from build123d import *

# Parameters (mm, degrees)
SKETCH3_R           = 2
BOSS_EXTRUDE1_DEPTH = 2.54
FILLET1_R           = 1
BOSS_EXTRUDE2_START = -2.54
BOSS_EXTRUDE2_DEPTH = 8.15
CUT_EXTRUDE1_DEPTH  = 68.045951128
CUT_EXTRUDE2_REACH  = 68.573
CUT_EXTRUDE3_REACH  = 68.573


with BuildPart() as part:
    # Sketch3 → Boss-Extrude1 (new body)
    with BuildSketch(Plane(origin=(0, 0, 0), x_dir=(1, 0, 0), z_dir=(0, 1, 0))):
        with BuildLine():
            Line((-10.5, 12.675), (-14.80167643, 18.402233616))
            ThreePointArc((-14.80167643, 18.402233616), (-17.462309014, 19.963696306), (-20.442771336, 19.167470316))
            Line((-20.442771336, 19.167470316), (-26.332078502, 14.625602737))
            ThreePointArc((-26.332078502, 14.625602737), (-27.469723987, 12.675134617), (-26.925, 10.483824754))
            Line((-26.925, 10.483824754), (-26.925, -10.483824754))
            ThreePointArc((-26.925, -10.483824754), (-27.469723987, -12.675134617), (-26.332078502, -14.625602737))
            Line((-26.332078502, -14.625602737), (-20.442771336, -19.167470316))
            ThreePointArc((-20.442771336, -19.167470316), (-17.462309014, -19.963696306), (-14.80167643, -18.402233616))
            Line((-14.80167643, -18.402233616), (-10.5, -12.675))
            Line((-10.5, -12.675), (10.5, -12.675))
            Line((10.5, -12.675), (14.80167643, -18.402233616))
            ThreePointArc((14.80167643, -18.402233616), (17.462309014, -19.963696306), (20.442771336, -19.167470316))
            Line((20.442771336, -19.167470316), (26.332078502, -14.625602737))
            ThreePointArc((26.332078502, -14.625602737), (27.469723987, -12.675134617), (26.925, -10.483824754))
            Line((26.925, -10.483824754), (26.925, 10.483824754))
            ThreePointArc((26.925, 10.483824754), (27.469723987, 12.675134617), (26.332078502, 14.625602737))
            Line((26.332078502, 14.625602737), (20.442771336, 19.167470316))
            ThreePointArc((20.442771336, 19.167470316), (17.462309014, 19.963696306), (14.80167643, 18.402233616))
            Line((14.80167643, 18.402233616), (10.5, 12.675))
            Line((10.5, 12.675), (-10.5, 12.675))
        make_face()
        with Locations(Location((-18, 16, 0), (0, 0, 270))):
            Circle(SKETCH3_R, mode=Mode.SUBTRACT)
        with Locations(Location((18, 16, 0), (0, 0, 270))):
            Circle(SKETCH3_R, mode=Mode.SUBTRACT)
        with Locations(Location((-18, -16, 0), (0, 0, 270))):
            Circle(SKETCH3_R, mode=Mode.SUBTRACT)
        with Locations(Location((18, -16, 0), (0, 0, 270))):
            Circle(SKETCH3_R, mode=Mode.SUBTRACT)
    extrude(amount=BOSS_EXTRUDE1_DEPTH)

    # Fillet1
    fillet1_edges = [part.edges().sort_by_distance(p)[0] for p in [
        (-26.925, 1.27, 10.483824754),
        (-26.925, 1.27, -10.483824754),
        (-10.5, 1.27, -12.675),
        (10.5, 1.27, -12.675),
        (26.925, 1.27, -10.483824754),
        (26.925, 1.27, 10.483824754),
        (10.5, 1.27, 12.675),
        (-10.5, 1.27, 12.675),
    ]]
    fillet(fillet1_edges, radius=FILLET1_R)

    # Sketch4 → Loft1 section 0
    with BuildSketch(Plane(origin=(0, 2.54, 0), x_dir=(1, 0, 0), z_dir=(0, 1, 0))):
        with BuildLine():
            Line((-26.925, -9), (-21.25, -12.675))
            Line((-21.25, -12.675), (21.25, -12.675))
            Line((21.25, -12.675), (26.925, -9))
            Line((26.925, -9), (26.925, 9))
            Line((26.925, 9), (21.25, 12.675))
            Line((21.25, 12.675), (-21.25, 12.675))
            Line((-21.25, 12.675), (-26.925, 9))
            Line((-26.925, 9), (-26.925, -9))
        make_face()
    # Sketch5 → Loft1 section 1
    with BuildSketch(Plane(origin=(0, 35, 0), x_dir=(1, 0, 0), z_dir=(0, 1, 0))):
        with BuildLine():
            Line((-17.75, -10.925), (17.75, -10.925))
            Line((17.75, -10.925), (25.2, -7.75))
            Line((25.2, -7.75), (25.2, 7.75))
            Line((25.2, 7.75), (17.75, 10.925))
            Line((17.75, 10.925), (-17.75, 10.925))
            Line((-17.75, 10.925), (-25.2, 7.75))
            Line((-25.2, 7.75), (-25.2, -7.75))
            Line((-25.2, -7.75), (-17.75, -10.925))
        make_face()
    loft()

    # Sketch7 → Boss-Extrude2 (add)
    with BuildSketch(Plane(origin=(0, 2.54, 0), x_dir=(1, 0, 0), z_dir=(0, 1, 0)).offset(BOSS_EXTRUDE2_START)):
        with BuildLine():
            Line((-22.124397263, -14.082078502), (-20.292318761, -11.706475765))
            Line((-20.292318761, -11.706475765), (-26.925, -6.591313823))
            Line((-26.925, -6.591313823), (-26.925, -10.183753403))
            ThreePointArc((-26.925, -10.183753403), (-26.961607557, -10.451848535), (-27.06875, -10.700315052))
            ThreePointArc((-27.06875, -10.700315052), (-26.19363735, -14.726205267), (-22.124397263, -14.082078502))
        make_face()
        with BuildLine():
            Line((-26.925, 10.183753403), (-26.925, 6.591313823))
            Line((-26.925, 6.591313823), (-20.292318761, 11.706475765))
            Line((-20.292318761, 11.706475765), (-22.124397263, 14.082078502))
            ThreePointArc((-22.124397263, 14.082078502), (-26.19363735, 14.726205267), (-27.06875, 10.700315052))
            ThreePointArc((-27.06875, 10.700315052), (-26.961607557, 10.451848535), (-26.925, 10.183753403))
        make_face()
        with BuildLine():
            Line((26.925, -10.183753403), (26.925, -6.591313823))
            Line((26.925, -6.591313823), (20.292318761, -11.706475765))
            Line((20.292318761, -11.706475765), (22.124397263, -14.082078502))
            ThreePointArc((22.124397263, -14.082078502), (26.19363735, -14.726205267), (27.06875, -10.700315052))
            ThreePointArc((27.06875, -10.700315052), (26.961607557, -10.451848535), (26.925, -10.183753403))
        make_face()
        with BuildLine():
            Line((22.124397263, 14.082078502), (20.292318761, 11.706475765))
            Line((20.292318761, 11.706475765), (26.925, 6.591313823))
            Line((26.925, 6.591313823), (26.925, 10.183753403))
            ThreePointArc((26.925, 10.183753403), (26.961607557, 10.451848535), (27.06875, 10.700315052))
            ThreePointArc((27.06875, 10.700315052), (26.19363735, 14.726205267), (22.124397263, 14.082078502))
        make_face()
    extrude(amount=BOSS_EXTRUDE2_DEPTH)

    # Sketch8 → Cut-Extrude1 (cut, through all)
    with BuildSketch(Plane(origin=(26.98377644, 1.433980726, 0), x_dir=(0, 0, -1), z_dir=(0.9985909302546928, 0.05306744777231502, 0))):
        Polygon((-9, 1.107579931), (9, 1.107579931), (7.75, 33.613382875), (-7.75, 33.613382875), align=None)
    cut_extrude1 = extrude(amount=CUT_EXTRUDE1_DEPTH, mode=Mode.SUBTRACT)

    # Sketch9 → Cut-Extrude2 (cut, up to next)
    with BuildSketch(Plane(origin=(23.985855334, 1.077940045, -5.108533277), x_dir=(-0.20789815344793566, -0.00934307914900991, -0.9781058555519203), z_dir=(0.9771196273503368, 0.04391239587739548, -0.20810798959926086)), mode=Mode.PRIVATE) as cut_extrude2_sk1:
        Polygon((-15.634592712, 6.932975266), (-14.203471003, 6.946359845), (-14.424341903, 1.328631852), align=None)
    cut_extrude2_tool1 = extrude(cut_extrude2_sk1.sketch, amount=CUT_EXTRUDE2_REACH, mode=Mode.PRIVATE) & part.part
    cut_extrude2 = cut_extrude2_tool1.solids().sort_by_distance((26.825624, 6.28, 9.322573))[0]
    add(cut_extrude2, mode=Mode.SUBTRACT)

    # Sketch10 → Cut-Extrude3 (cut, up to next)
    with BuildSketch(Plane(origin=(23.985855334, 1.077940045, 5.108533278), x_dir=(0.2078981534584427, 0.009343079149391592, -0.9781058555496834), z_dir=(0.9771196273481212, 0.04391239587687057, 0.20810798960977442)), mode=Mode.PRIVATE) as cut_extrude3_sk1:
        Polygon((14.424341903, 1.328631852), (15.634592712, 6.932975266), (14.203471003, 6.946359845), align=None)
    cut_extrude3_tool1 = extrude(cut_extrude3_sk1.sketch, amount=CUT_EXTRUDE3_REACH, mode=Mode.PRIVATE) & part.part
    cut_extrude3 = cut_extrude3_tool1.solids().sort_by_distance((26.825624, 6.28, -9.322573))[0]
    add(cut_extrude3, mode=Mode.SUBTRACT)

    # Mirror1: Cut-Extrude1, Cut-Extrude2, Cut-Extrude3 across plane
    add(cut_extrude1.mirror(Plane(origin=(0, 0, 0), x_dir=(0, 0, 1), z_dir=(1, 0, 0))), mode=Mode.SUBTRACT)
    add(cut_extrude2.mirror(Plane(origin=(0, 0, 0), x_dir=(0, 0, 1), z_dir=(1, 0, 0))), mode=Mode.SUBTRACT)
    add(cut_extrude3.mirror(Plane(origin=(0, 0, 0), x_dir=(0, 0, 1), z_dir=(1, 0, 0))), mode=Mode.SUBTRACT)


solid = part.part
The listing builds one solid part. Answer for the finished solid, in the listing's coordinates (mm). A direction names the side the tool comes from. Give positions to 0.01 mm unless a question says otherwise; leave off trailing zeros. Write each loop counter-clockwise with the first axis right and the second up, starting at its lowest first coordinate (ties: lowest second). Pieces come first, ordered by that corner, then holes. Notation, with made-up numbers: (38.25, 88) -> (69.25, 88) arc R4 cw to (69.25, 95) -> close; hole circle Ø3 at (80, 43.5). An arc over 180 degrees is marked (long way). Use a Markdown table: item, result.
(1) Section B-B, the plane z = 3.5 is taken. Determine the outline of the cut face in (x, y) (3 decimals), then the cut area to 3 significant figures.
Return value:
| item | result |
|---|---|
| outline | (-26.925, 0) -> (26.925, 0) -> (26.925, 2.54) -> (25.2, 35) -> (-25.2, 35) -> (-26.925, 2.54) -> close |
| area | 1,830 mm2 |
(2) Find the intervals of material crossed by probe 1 along X at (y, z) = (0.8, 16); probe 2 along Y at (x, z) = (-14, 17); probe 3 along Z at (x, y) = (-2.5, 17.5), in increasing order. Write a range as from..to.
Return value:
| item | result |
|---|---|
| probe 1 | -24.55..-20, -16..-13, 13..16, 20..24.55 |
| probe 2 | 0..2.54 |
| probe 3 | -11.87..11.87 |
(3) Section A-A, the plane z = -16 is taken. Determine the outline of the cut face in (x, y).
Return value:
| item | result |
|---|---|
| outline | (-24.55, 0) -> (-20, 0) -> (-20, 2.54) -> (-24.55, 2.54) -> close; (-16, 0) -> (-13, 0) -> (-13, 2.54) -> (-16, 2.54) -> close; (13, 0) -> (16, 0) -> (16, 2.54) -> (13, 2.54) -> close; (20, 0) -> (24.55, 0) -> (24.55, 2.54) -> (20, 2.54) -> close |
(4) Flat-ended cylindrical pins translate along their axes: P1, Ø2, axis at x = -17, z = -16.5, coming from the +Y side; P2, Ø5, axis at x = -18, z = -16, coming from the -Y side; P3, Ø5, axis at y = 26.5, z = -1.5, coming from the -X side; P4, Ø6.5, axis at y = 5, z = -5, coming from the -X side (3 decimals). Find the tip coordinate at first contact, or state that the pin passes through.
Return value:
| item | result |
|---|---|
| P1 | y = 2.54 |
| P2 | y = 0 |
| P3 | x = -25.78 |
| P4 | x = -26.925 |
(5) Section C-C, the plane x = -19 is taken. Give the number of separate pieces and of enclosed holes in the cut face, then the cut area to 3 significant figures.
Return value:
| item | result |
|---|---|
| separate pieces | 3 |
| enclosed holes | 0 |
| area | 843 mm2 |
(6) Determine the mould class of faces 1 (the flat face through (-23.346, 1.252, -16.928)), 2 (the flat face through (0, 0, 0)), 3 (the flat face through (-16, 2.54, 15)) for opening direction X: released by +X, released by -X, zero draft, split by the parting line, or undercut.
Return value:
| item | result |
|---|---|
| face 1 | released by -X |
| face 2 | zero draft |
| face 3 | undercut |
(7) For faces 4 (the flat face through (0, 1, 12.675)), 5 (the flat face through (25, 8.15, -13)), 6 (the flat face through (-21.45, 5.31, 13.21)), determine the directions among +Z, -Z, +X, -X, +Y, -Y from which every point of the face is accessible in a straight line to the end or side of a thin tool.
Return value:
| item | result |
|---|---|
| face 4 | +Z, +Y, -Y |
| face 5 | -Z, +X, +Y |
| face 6 | +Z, +Y |
